Can you work these out from the model? Positions are in its coordinate system, mm. A direction names the side the tool comes from. Round coordinates to 2 decimals unless told otherwise and drop trailing zeros. Loops run counter-clockwise (first coordinate to the right, second up) from the corner with the lowest first, then second, coordinate; pieces in that order, holes last. Notation, with made-up numbers: (13, -14.5) -> (38, -14.5) arc R6 cw to (38, -4.5) -> close; hole circle Ø6 at (5, 26). An arc over 180 degrees is marked (long way). Use a Markdown table: item, result.
Autodesk Inventor part; units mm, degrees
ref_plane "YZ Plane" through (0, 0, 0) normal (1, 0, 0) x (0, 1, 0)
ref_plane "XZ Plane" through (0, 0, 0) normal (0, 1, 0) x (-1, 0, 0)
ref_plane "XY Plane" through (0, 0, 0) normal (0, 0, 1) x (1, 0, 0)
sketch "Sketch1" plane through (0, 0, 0) normal (0, 0, 1) x (1, 0, 0)
  line L0 (-12.7, 10.16) -> (0, 10.16)
  line L1 (0, 10.16) -> (0, 0)
  line L2 (0, 0) -> (1.27, 0)
  line L3 (1.27, 0) -> (1.27, -6.35)
  line L4 (1.27, -6.35) -> (-0.0109, -6.35)
  line L5 (-0.0109, -6.35) -> (-12.7, -6.35)
  line L6 (-12.7, -6.35) -> (-12.7, 10.16)
  dimension "d0" = 12.7
  dimension "d1" = 1.27
  dimension "d2" = 6.35
  dimension "d3" = 16.51
extrude "Extrusion1" add sketch "Sketch1" along normal blind 9.525
hole "Hole1" at (-6.35, 3.81, 9.525) direction (0, 0, -1) diameter 3.556 end through all
hole "Hole2" at (-12.7, -4.445, 2.54) direction (1, 0, 0) diameter 1.6002 end through all
hole "Hole3" at (-12.7, -2.667, 2.54) direction (1, 0, 0) diameter 1.6002 depth 25.4 tip angle 118
hole "Hole4" at (-12.7, -2.667, 6.985) direction (1, 0, 0) diameter 1.6002 end through all
hole "Hole5" at (-12.7, -4.445, 6.985) direction (1, 0, 0) diameter 1.6002 end through all
sketch "Sketch2" plane through (1.27, -6.35, 0) normal (1, 0, 0) x (0, 0, -1)
  circle A0 centre (-6.985, 1.905) radius 0.8001
  circle A1 centre (-6.985, 3.683) radius 0.8001
  circle A2 centre (-2.54, 3.683) radius 0.8001
  circle A3 centre (-2.54, 1.905) radius 0.8001
  arc A4 (-5.2178, 3.683) -> (-8.7522, 3.683) centre (-6.985, 3.683) ccw
  line L0 (-8.7522, 3.683) -> (-8.7522, 1.905)
  arc A5 (-8.7522, 1.905) -> (-5.2178, 1.905) centre (-6.985, 1.905) ccw
  line L1 (-5.2178, 1.905) -> (-5.2178, 3.683)
  line L2 (-4.3207, 3.683) -> (-4.3207, 1.905)
  arc A6 (-4.3207, 1.905) -> (-0.7593, 1.905) centre (-2.54, 1.905) ccw
  line L3 (-0.7593, 1.905) -> (-0.7593, 3.683)
  arc A7 (-0.7593, 3.683) -> (-4.3207, 3.683) centre (-2.54, 3.683) ccw
extrude "Extrusion3" add sketch "Sketch2" along normal blind 5.08
properties part number "lickport_DHO_v0"
1. If we mould it in two halves opening along Z, with no side actions, what happens to faces 1 (the flat face through (1.27, -2, 5)), 2 (the flat face through (-12.7, 2, 5)), 3 (the flat face through (-7.4, 2, 0))? For each: +Z half, -Z half, draft (parallel to the pull), parting line (faces both ways), or undercut.
Answer sheet:
| item | result |
|---|---|
| face 1 | undercut |
| face 2 | draft |
| face 3 | -Z half |
2. I want a section at B-B (y = 3.81). Please give me the cut outline in (x, z) (3 decimals), plus the area to 3 significant figures.
Answer sheet:
| item | result |
|---|---|
| outline | (-12.7, 0) -> (-8.128, 0) -> (-8.128, 9.525) -> (-12.7, 9.525) -> close; (-4.572, 0) -> (0, 0) -> (0, 9.525) -> (-4.572, 9.525) -> close |
| area | 87.1 mm² |
3. I need wall thicknesses on line 1 (Y direction, x = 4.25, z = 2.54); line 2 (Y direction, x = -4, z = 2.5); line 3 (Z direction, x = -9, y = -4.5) (3 decimals). Which ranges of each line are inside material? Lowest first, please.
Answer sheet:
| item | result |
|---|---|
| line 1 | y = -6.23 to -5.25, -3.64 to -3.47, -1.87 to -0.89 |
| line 2 | y = -6.35 to -5.24, -3.65 to -3.47, -1.87 to 10.16 |
| line 3 | z = 0 to 1.742, 3.338 to 6.187, 7.783 to 9.525 |
4. Will these pins go through, and if not, where does the flat tip stop? pin 1 Ø1.4 at (x, y) = (4.5, -4) entering from -Z; pin 2 Ø0.5 at (x, y) = (4.5, -3) entering from +Z.
Answer sheet:
| item | result |
|---|---|
| pin 1 | stops at z = 0.76 |
| pin 2 | stops at z = 8.75 |
5. I want a section at A-A (x = 1.75). Please give me the cut outline in (y, z) (3 decimals), plus the area to 3 significant figures.
Answer sheet:
| item | result |
|---|---|
| outline | (-4.445, 0.759) -> (-2.667, 0.759) arc R1.781 ccw to (-2.667, 4.321) -> (-4.445, 4.321) arc R1.781 ccw to start; (-4.445, 5.218) -> (-2.667, 5.218) arc R1.767 ccw to (-2.667, 8.752) -> (-4.445, 8.752) arc R1.767 ccw to start; hole circle Ø1.6 at (-4.445, 2.54); hole circle Ø1.6 at (-4.445, 6.985); hole circle Ø1.6 at (-2.667, 2.54); hole circle Ø1.6 at (-2.667, 6.985) |
| area | 24.3 mm² |
6. I want a section at D-D (y = -4). Please give me the cut outline in (x, z) (3 decimals), plus the area to 3 significant figures.
Answer sheet:
| item | result |
|---|---|
| outline | (-12.7, 0) -> (1.27, 0) -> (1.27, 0.759) -> (6.35, 0.759) -> (6.35, 1.875) -> (-12.7, 1.875) -> close; (-12.7, 3.205) -> (6.35, 3.205) -> (6.35, 4.321) -> (1.27, 4.321) -> (1.27, 5.218) -> (6.35, 5.218) -> (6.35, 6.32) -> (-12.7, 6.32) -> close; (-12.7, 7.65) -> (6.35, 7.65) -> (6.35, 8.752) -> (1.27, 8.752) -> (1.27, 9.525) -> (-12.7, 9.525) -> close |
| area | 118 mm² |
7. Which directions (+Z, -Z, +X, -X, +Y, -Y) give clear straight access to the entire face, cutting with the end or side of a thin tool? Please do faces 4 (the cylindrical face through (3.8, -0.9, 7)), 5 (the flat face through (4, -4, 5.218)), 6 (the flat face through (1, 0, 5)), 7 (the cylindrical face through (3.774, -6.225, 2.501)), 8 (the flat face through (4, -4, 8.752)).
Answer sheet:
| item | result |
|---|---|
| face 4 | +X, +Y |
| face 5 | +X, +Y, -Y |
| face 6 | +Z, -Z, +X, +Y |
| face 7 | +X, -Y |
| face 8 | +Z, +X, +Y, -Y |
8. I want a section at C-C (z = 2.54). Please give me the cut outline in (x, y), plus the area to 3 significant figures.
Answer sheet:
| item | result |
|---|---|
| outline | (-12.7, -6.35) -> (1.27, -6.35) -> (1.27, -6.23) -> (6.35, -6.23) -> (6.35, -5.25) -> (-12.7, -5.25) -> close; (-12.7, -3.64) -> (6.35, -3.64) -> (6.35, -3.47) -> (-12.7, -3.47) -> close; (-12.7, -1.87) -> (6.35, -1.87) -> (6.35, -0.89) -> (1.27, -0.89) -> (1.27, 0) -> (0, 0) -> (0, 10.16) -> (-12.7, 10.16) -> close; hole circle Ø3.56 at (-6.35, 3.81) |
| area | 174 mm² |
